from build123d import *

# Parameters (mm, degrees)
F0_R          = 2.3
F1_DEPTH      = 13
F3_DEPTH      = 46
F6_DEPTH      = 52.2
F8_DEPTH      = 25
F10_DEPTH     = 25
F11_T1_DEPTH  = 69.4664340584
F11_T3_DEPTH  = 69.4664340584
F11_T8_DEPTH  = 31.9524083705
F11_T13_DEPTH = 31.9524083705
F11_T19_DEPTH = 31.9524083705
F11_T23_DEPTH = 31.9524083705
F15_DEPTH     = 5
F16_DEPTH     = 5
F18_R         = 3.2
F19_DEPTH     = 28


# Not quite as in the source:
# - a fillet or chamfer that OpenCascade refuses, or shapes differently, is made with other operations: its cross-section is extruded or revolved along the edge and cut away or added
# - a feature names something its author has since deleted; it is built from what else it names


with BuildPart() as f1:
    # F0 (on Front) → F1 (new body)
    with BuildSketch(Plane.XZ):
        Polygon((10, 40), (-10, 40), (-17.9806351662, -11.8325809017), (-8.0368565166, -18.5498173996), (0, -8.6111112242), (8.0368565166, -18.5498173996), (17.9806351662, -11.8325809017), align=None)
        with Locations((-12, 0)):
            Circle(F0_R, mode=Mode.SUBTRACT)
        with Locations((12, 0)):
            Circle(F0_R, mode=Mode.SUBTRACT)
    extrude(amount=-F1_DEPTH)

    # F2 (on face) → F3 (cut)
    with BuildSketch(Plane.XY.offset(40)):
        with BuildLine():
            Line((-8, 0), (8, 0))
            ThreePointArc((8, 0), (0, 8), (-8, 0))
        make_face()
    extrude(amount=-F3_DEPTH, mode=Mode.SUBTRACT)

    # F5 (on offset) → F6 (cut)
    with BuildSketch(Plane.YZ.offset(25)):
        Polygon((13, -3.9485500787), (4.1381944902, -18.5498173996), (13, -18.5498173996), align=None)
    extrude(amount=-F6_DEPTH, mode=Mode.SUBTRACT)

    # F7 (on face) → F8 (cut)
    with BuildSketch(Plane(origin=(-11.122658813, 0, -16.4652915326), x_dir=(0.8286482208, 0, -0.5597697082), z_dir=(-0.5597697082, 0, -0.8286482208))):
        with BuildLine():
            ThreePointArc((-6.8761009811, 0), (-2.2761009811, -4.6), (2.3238990189, 0))
            Line((2.3238990189, 0), (-6.8761009811, 0))
        make_face()
    extrude(amount=-F8_DEPTH, mode=Mode.SUBTRACT)

    # F9 (on face) → F10 (cut)
    with BuildSketch(Plane(origin=(11.122658813, 0, -16.4652915326), x_dir=(0.8286482208, 0, 0.5597697082), z_dir=(0.5597697082, 0, -0.8286482208))):
        with BuildLine():
            ThreePointArc((-2.3238990189, 0), (2.2761009811, -4.6), (6.8761009811, 0))
            Line((6.8761009811, 0), (-2.3238990189, 0))
        make_face()
    extrude(amount=-F10_DEPTH, mode=Mode.SUBTRACT)

    # F11: fillet of radius 5 on 4 edges, made by hand

    # F11_s2 → F11_t1 (cut)
    with BuildSketch(Plane(origin=(7.6867833124, 0, 49.9240736631), x_dir=(0, 1, 0), z_dir=(-0.152176248, 0, -0.9883533728))):
        with BuildLine():
            ThreePointArc((13, -10.9705836466), (11.5355339059, -14.5061175525), (8, -15.9705836466))
            Line((8, -15.9705836466), (13, -15.9705836466))
            Line((13, -15.9705836466), (13, -10.9705836466))
        make_face()
    extrude(amount=F11_T1_DEPTH, mode=Mode.SUBTRACT)

    # F11_s4 → F11_t3 (cut)
    with BuildSketch(Plane(origin=(2.8843579817, 0, -18.733310736), x_dir=(0, 1, 0), z_dir=(-0.152176248, 0, 0.9883533728))):
        with BuildLine():
            ThreePointArc((8, -15.9705836466), (11.5355339059, -14.5061175525), (13, -10.9705836466))
            Line((13, -10.9705836466), (13, -15.9705836466))
            Line((13, -15.9705836466), (8, -15.9705836466))
        make_face()
    extrude(amount=F11_T3_DEPTH, mode=Mode.SUBTRACT)


with BuildPart() as f11_tool6:
    # F11_s7 → F11_t8 (new body)
    with BuildSketch(Plane(origin=(4.0911710208, 3.0705977915, 5.0593097692), x_dir=(0.6002776597, -0.7997916799, 0), z_dir=(-0.5686414, -0.4267895471, -0.7032052622))):
        with BuildLine():
            ThreePointArc((-10.7347001393, -7.9787789452), (-7.9821654916, -9.2854915519), (-4.9822833283, -8.7519638303))
            Line((-4.9822833283, -8.7519638303), (-8.1340389445, -10.4154145762))
            Line((-8.1340389445, -10.4154145762), (-10.7347001393, -7.9787789452))
        make_face()
    extrude(amount=F11_T8_DEPTH)

    split(bisect_by=Plane(origin=(-4.2102294585, 0, -3.404568911), x_dir=(0, 1, 0), z_dir=(-0.7775800359, 0, -0.6287839754)), keep=Keep.TOP)


with BuildPart() as f1_1:
    add(f1.part)

    # F11_t5: cut F11_tool6
    add(f11_tool6.part, mode=Mode.SUBTRACT)


with BuildPart() as f11_tool11:
    # F11_s12 → F11_t13 (new body)
    with BuildSketch(Plane(origin=(14.0782912081, -10.566356105, -17.4097919354), x_dir=(-0.6002776597, -0.7997916799, 0), z_dir=(-0.5686414, 0.4267895471, 0.7032052622))):
        with BuildLine():
            ThreePointArc((-10.7347001393, -7.9787789452), (-7.9821654916, -9.2854915519), (-4.9822833283, -8.7519638303))
            Line((-4.9822833283, -8.7519638303), (-8.1340389445, -10.4154145762))
            Line((-8.1340389445, -10.4154145762), (-10.7347001393, -7.9787789452))
        make_face()
    extrude(amount=F11_T13_DEPTH)

    split(bisect_by=Plane(origin=(4.2102294585, 0, -3.404568911), x_dir=(0, 1, 0), z_dir=(0.7775800359, 0, -0.6287839754)), keep=Keep.TOP)


with BuildPart() as f1_2:
    add(f1_1.part)

    # F11_t10: cut F11_tool11
    add(f11_tool11.part, mode=Mode.SUBTRACT)


with BuildPart() as f11_tool17:
    # F11_s18 → F11_t19 (new body)
    with BuildSketch(Plane(origin=(14.0782912081, -10.566356105, -17.4097919354), x_dir=(-0.6002776597, -0.7997916799, 0), z_dir=(-0.5686414, 0.4267895471, 0.7032052622))):
        with BuildLine():
            ThreePointArc((-10.7347001393, -7.9787789452), (-7.9821654916, -9.2854915519), (-4.9822833283, -8.7519638303))
            Line((-4.9822833283, -8.7519638303), (-8.1340389445, -10.4154145762))
            Line((-8.1340389445, -10.4154145762), (-10.7347001393, -7.9787789452))
        make_face()
    extrude(amount=F11_T19_DEPTH)

    split(bisect_by=Plane(origin=(4.2102294585, 0, -3.404568911), x_dir=(0, 1, 0), z_dir=(-0.7775800359, 0, 0.6287839754)), keep=Keep.TOP)


with BuildPart() as f11_tool21:
    # F11_s22 → F11_t23 (new body)
    with BuildSketch(Plane(origin=(4.0911710208, 3.0705977915, 5.0593097692), x_dir=(0.6002776597, -0.7997916799, 0), z_dir=(-0.5686414, -0.4267895471, -0.7032052622))):
        with BuildLine():
            ThreePointArc((-10.7347001393, -7.9787789452), (-7.9821654916, -9.2854915519), (-4.9822833283, -8.7519638303))
            Line((-4.9822833283, -8.7519638303), (-8.1340389445, -10.4154145762))
            Line((-8.1340389445, -10.4154145762), (-10.7347001393, -7.9787789452))
        make_face()
    extrude(amount=F11_T23_DEPTH)

    split(bisect_by=Plane(origin=(-4.2102294585, 0, -3.404568911), x_dir=(0, 1, 0), z_dir=(0.7775800359, 0, 0.6287839754)), keep=Keep.TOP)


with BuildPart() as f11_tool17_1:
    add(f11_tool17.part)

    # F11_t25: intersect F11_tool21
    add(f11_tool21.part, mode=Mode.INTERSECT)


with BuildPart() as f1_3:
    add(f1_2.part)

    # F11_t15: cut F11_tool17
    add(f11_tool17_1.part, mode=Mode.SUBTRACT)

    # F14 (on face) → F15 (cut)
    with BuildSketch(Plane.XZ):
        Polygon((-15.1459260242, -6.5643846345), (-10, 1.0533238305), (-10, 26.8573445146), align=None)
    extrude(amount=-F15_DEPTH, mode=Mode.SUBTRACT)

    # F12 (on face) → F16 (cut)
    with BuildSketch(Plane.XZ):
        Polygon((15.1459253956, -6.5643830302), (10.0000003771, 26.8573395869), (10.0000003771, 1.0533239459), align=None)
    extrude(amount=-F16_DEPTH, mode=Mode.SUBTRACT)

    # F18 (on offset) → F19 (cut)
    with BuildSketch(Plane(origin=(0, 38, 0), x_dir=(-1, 0, 0), z_dir=(0, 1, 0))):
        with Locations((-12, 0)):
            Circle(F18_R)
        with Locations((12, 0)):
            Circle(F18_R)
    extrude(amount=-F19_DEPTH, mode=Mode.SUBTRACT)


solid = f1_3.part
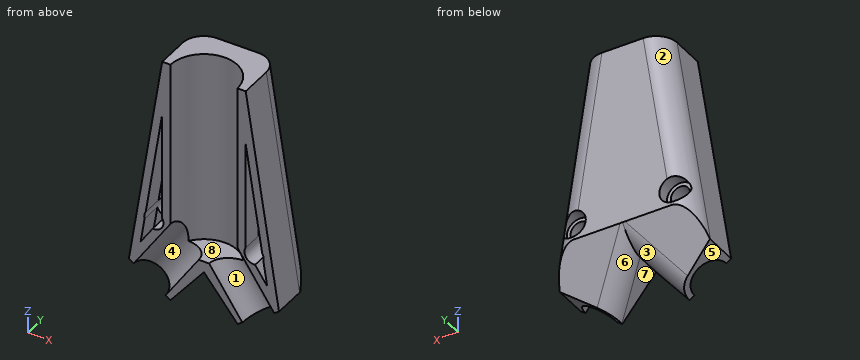
Read the model definition and answer for the solid it produces. Units are mm, in the model's axes. Face numbers are marked on the shaded views. A direction names the side the tool comes from. Coordinates: 2 decimals unless noted, no trailing zeros. Answer in a Markdown table with one row per item.
Item 1: For the marked faces 5, 6, 7 and 8, determine the directions among +Z, -Z, +X, -X, +Y, -Y from which every point of the face is accessible in a straight line to the end or side of a thin tool.
Returned:
| item | result |
|---|---|
| face 5 | -Z, -X, +Y, -Y |
| face 6 | -Z, +Y |
| face 7 | -Z, +Y, -Y |
| face 8 | +Z, -Y |
Item 2: A cutting plane is placed at A-A on y = 3.75. Give the number of separate pieces and of enclosed holes in the cut face, plus the area to 3 significant figures.
Returned:
| item | result |
|---|---|
| separate pieces | 3 |
| enclosed holes | 2 |
| area | 618 mm^2 |
Item 3: For a pull along Z with two mould halves and no side action, classify the marked faces 1, 2, 3 and 4 as released by +Z, released by -Z, zero draft, split by the parting line, or undercut.
Returned:
| item | result |
|---|---|
| face 1 | undercut |
| face 2 | released by +Z |
| face 3 | released by -Z |
| face 4 | undercut |
Item 4: Straight lines are drawn through the part: line 1 along X through (y, z) = (4, 0); line 2 along X through (y, z) = (5.5, 0); line 3 along X through (y, z) = (10.25, 31). For each, find the intervals that lie inside material, in ascending order. Write a range as [from, to].
Returned:
| item | result |
|---|---|
| line 1 | x = [-16.16, -14.3], [-9.7, -6.93], [6.93, 9.7], [14.3, 16.16] |
| line 2 | x = [-16.16, -14.3], [-9.7, -5.81], [5.81, 9.7], [14.3, 16.16] |
| line 3 | x = [-10.84, 10.84] |
Item 5: Each of these flat-tipped pins is pushed along its axis until it touches: P1, Ø5.5, axis at y = 3.5, z = 17, coming from the +X side; P2, Ø6, axis at y = 5, z = 28, coming from the -X side; P3, Ø6, axis at x = 12, z = 0, coming from the +Y side; P4, Ø4, axis at x = 12, z = 0, coming from the -Y side. Where does it stop, or does it pass through?
Returned:
| item | result |
|---|---|
| P1 | stops at x = 13.96 |
| P2 | stops at x = -12.31 |
| P3 | stops at y = 10 |
| P4 | passes through |
